Build history of the part. All positions in model axes, mm. Give positions to 0.01 mm unless a question says otherwise; leave off trailing zeros. Order: outer loops, then holes, each group sorted by start corner. A loop starts at its lowest first (then second) coordinate and runs counter-clockwise, first axis right, second up. Notation, with made-up numbers: M -29,85.25 L -21,85.25 A24 ccw -21,111.25 Z; hole C 87.25,53 d5. An arc over 180 degrees is marked long. One line per item, written item: value.
from build123d import *

# Parameters (mm, degrees)
PAD001_DEPTH            = 45.961941
PAD_DEPTH               = 45.961941
CYLINDER002_R           = 40
CYLINDER002_DEPTH       = 130
CYLINDER002_PITCH_ANGLE = 90
CYLINDER001_R           = 40
CYLINDER001_DEPTH       = 130
CYLINDER001_ROLL_ANGLE  = 90
CYLINDER_R              = 40
CYLINDER_DEPTH          = 130
BOX001_W                = 120
BOX001_H                = 120
BOX001_DEPTH            = 120
BOX_W                   = 130
BOX_H                   = 130
BOX_DEPTH               = 130


with BuildPart() as pad001:
    # Sketch001 → Pad001 (new body, symmetric)
    with BuildSketch(Plane(origin=(0, 0, 0), x_dir=(-0.707107, 0.707107, 0), z_dir=(0.707107, 0.707107, 0))):
        Polygon((-100, 10), (-100, 85), (-25, 85), align=None)
        Polygon((25, 85), (100, 85), (100, 10), align=None)
        Polygon((25, -85), (100, -85), (100, -10), align=None)
        Polygon((-100, -10), (-100, -85), (-25, -85), align=None)
    extrude(amount=PAD001_DEPTH, both=True)


with BuildPart() as pad:
    # Sketch → Pad (new body, symmetric)
    with BuildSketch(Plane(origin=(0, 0, 0), x_dir=(0.707107, 0.707107, 0), z_dir=(0.707107, -0.707107, 0))):
        Polygon((-100, 10), (-100, 85), (-25, 85), align=None)
        Polygon((25, 85), (100, 85), (100, 10), align=None)
        Polygon((25, -85), (100, -85), (100, -10), align=None)
        Polygon((-100, -10), (-100, -85), (-25, -85), align=None)
    extrude(amount=PAD_DEPTH, both=True)


with BuildPart() as cylinder002:
    # Cylinder002 → Cylinder002 (new body)
    with BuildSketch(Plane.XY):
        Circle(CYLINDER002_R)
    extrude(amount=CYLINDER002_DEPTH)


with BuildPart() as cylinder002_1:
    # Cylinder002 pitch: moved
    add(cylinder002.part.rotate(Axis((0, 0, 0), (0, 1, 0)), CYLINDER002_PITCH_ANGLE))


with BuildPart() as cylinder002_2:
    # Cylinder002 placement: moved
    add(cylinder002_1.part.moved(Location((-65, 0, 0))))


with BuildPart() as cylinder001:
    # Cylinder001 → Cylinder001 (new body)
    with BuildSketch(Plane.XY):
        Circle(CYLINDER001_R)
    extrude(amount=CYLINDER001_DEPTH)


with BuildPart() as cylinder001_1:
    # Cylinder001 roll: moved
    add(cylinder001.part.rotate(Axis((0, 0, 0), (1, 0, 0)), CYLINDER001_ROLL_ANGLE))


with BuildPart() as cylinder001_2:
    # Cylinder001 placement: moved
    add(cylinder001_1.part.moved(Location((0, 65, 0))))


with BuildPart() as cylinder:
    # Cylinder → Cylinder (new body)
    with BuildSketch(Plane.XY.offset(-65)):
        Circle(CYLINDER_R)
    extrude(amount=CYLINDER_DEPTH)


with BuildPart() as cube001:
    # Box001 → Box001 (new body)
    with BuildSketch(Plane(origin=(-60, -60, -60), x_dir=(1, 0, 0), z_dir=(0, 0, 1))):
        with Locations((60, 60)):
            Rectangle(BOX001_W, BOX001_H)
    extrude(amount=BOX001_DEPTH)


with BuildPart() as cut005:
    # Box → Box (new body)
    with BuildSketch(Plane(origin=(-65, -65, -65), x_dir=(1, 0, 0), z_dir=(0, 0, 1))):
        with Locations((65, 65)):
            Rectangle(BOX_W, BOX_H)
    extrude(amount=BOX_DEPTH)

    # Cut: cut Cube001
    add(cube001.part, mode=Mode.SUBTRACT)

    # Cut001: cut Cylinder
    add(cylinder.part, mode=Mode.SUBTRACT)

    # Cut002: cut Cylinder001
    add(cylinder001_2.part, mode=Mode.SUBTRACT)

    # Cut003: cut Cylinder002
    add(cylinder002_2.part, mode=Mode.SUBTRACT)

    # Cut004: cut Pad
    add(pad.part, mode=Mode.SUBTRACT)

    # Cut005: cut Pad001
    add(pad001.part, mode=Mode.SUBTRACT)


solid = cut005.part
1) Pin check, flat tip, straight feed: pin 1 (8 mm diameter, centred on x = 9, z = 33.5, fed in from -Y). Stop position of the tip, or through.
Check values:
pin 1: through
2) Saw through at D-D, the plane y = -7. Write the cut outline in (x, z).
Check values:
outline: M -65,-59.09 L -56.64,-65 L -39.38,-65 L -39.38,-60 L -60,-60 L -60,-39.38 L -65,-39.38 Z; M -65,39.38 L -60,39.38 L -60,60 L -39.38,60 L -39.38,65 L -56.64,65 L -65,59.09 Z; M 39.38,-65 L 56.64,-65 L 65,-59.09 L 65,-39.38 L 60,-39.38 L 60,-60 L 39.38,-60 Z; M 39.38,60 L 60,60 L 60,39.38 L 65,39.38 L 65,59.09 L 56.64,65 L 39.38,65 Z
3) Mould opens along Z. For faces 1 (the face through (-29, 29, 65)), 2 (the face through (-1, 41, -60)), 3 (the face through (-37.07, -32.559, -60.765)), 4 (the face through (-1, 41, 60)) say: released by +Z, released by -Z, zero draft, split by the parting line, or undercut.
Check values:
face 1: released by +Z
face 2: undercut
face 3: released by -Z
face 4: undercut
4) Saw through at B-B, the plane x = -35.5. Give the number of separate pieces and of enclosed holes in the cut face, then the cut area to 3 significant figures.
Check values:
separate pieces: 8
enclosed holes: 0
area: 710 mm^2
5) Drill centre line: probe 1 along Y at (x, z) = (39.5, 19.5). Where is it in solid material? Low to high. Write a range as from..to.
Check values:
probe 1: -65..-60, 60..65
6) Saw through at A-A, the plane z = 0. Write the cut outline in (x, y).
Check values:
outline: M -65,-65 L -40,-65 L -40,-60 L -60,-60 L -60,-40 L -65,-40 Z; M -65,40 L -60,40 L -60,60 L -40,60 L -40,65 L -65,65 Z; M 40,-65 L 65,-65 L 65,-40 L 60,-40 L 60,-60 L 40,-60 Z; M 40,60 L 60,60 L 60,40 L 65,40 L 65,65 L 40,65 Z
